```python
from build123d import *

# Parameters (mm, degrees)
BOSS_EXTRUDE1_DEPTH = 3
SKETCH3_W           = 4.2
SKETCH3_H           = 3.2
SKETCH3_W_2         = 3.2
SKETCH3_H_2         = 8.2
SKETCH3_W_3         = 8.2
CUT_EXTRUDE1_DEPTH  = 4


with BuildPart() as part:
    # Sketch1 → Boss-Extrude1 (new body)
    with BuildSketch(Plane.XY):
        Polygon((0, 52.125), (80, 52.125), (80, 3.175), (64, 3.175), (64, 15.625), (16, 15.625), (16, 3.175), (0, 3.175), align=None)
    extrude(amount=-BOSS_EXTRUDE1_DEPTH)

    # Sketch3 → Cut-Extrude1 (cut, through all)
    with BuildSketch(Plane.XY):
        with Locations((2, 50.625)):
            Rectangle(SKETCH3_W, SKETCH3_H)
        with Locations((1.5, 20.925)):
            Rectangle(SKETCH3_W_2, SKETCH3_H_2)
        with Locations((24, 17.125)):
            Rectangle(SKETCH3_W_3, SKETCH3_H)
        with Locations((40, 17.125)):
            Rectangle(SKETCH3_W_3, SKETCH3_H)
        with Locations((1.5, 36.925)):
            Rectangle(SKETCH3_W_2, SKETCH3_H_2)
        with Locations((40, 50.625)):
            Rectangle(SKETCH3_W_3, SKETCH3_H)
        with Locations((40, 42.425)):
            Rectangle(SKETCH3_W_3, SKETCH3_H)
        with Locations((24, 42.425)):
            Rectangle(SKETCH3_W_3, SKETCH3_H)
        with Locations((24, 50.625)):
            Rectangle(SKETCH3_W_3, SKETCH3_H)
        with Locations((56, 42.425)):
            Rectangle(SKETCH3_W_3, SKETCH3_H)
        with Locations((56, 17.125)):
            Rectangle(SKETCH3_W_3, SKETCH3_H)
        with Locations((78.5, 36.925)):
            Rectangle(SKETCH3_W_2, SKETCH3_H_2)
        with Locations((78, 50.625)):
            Rectangle(SKETCH3_W, SKETCH3_H)
        with Locations((78.5, 20.925)):
            Rectangle(SKETCH3_W_2, SKETCH3_H_2)
        with Locations((56, 50.625)):
            Rectangle(SKETCH3_W_3, SKETCH3_H)
        Polygon((76.9, 9.025), (76.9, 6.275), (67.9, 6.275), (67.9, 3.075), (80.1, 3.075), (80.1, 9.025), align=None)
        Polygon((3.1, 6.275), (3.1, 9.025), (-0.1, 9.025), (-0.1, 3.075), (12.1, 3.075), (12.1, 6.275), align=None)
    extrude(amount=-CUT_EXTRUDE1_DEPTH, mode=Mode.SUBTRACT)


solid = part.part
```
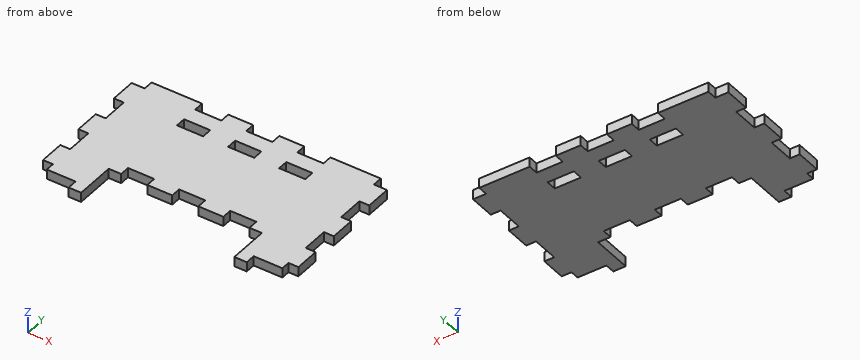
Read the model definition and answer for the solid it produces. Units are mm, in the model's axes. Give positions to 0.01 mm unless a question says otherwise; leave off trailing zeros. Order: outer loops, then holes, each group sorted by start corner. A loop starts at its lowest first (then second) coordinate and runs counter-clockwise, first axis right, second up. Notation, with made-up numbers: (45.5, 7) -> (52.5, 7) arc R25 cw to (52.5, 44) -> close; hole circle Ø7 at (-37.5, -17.75). An arc over 180 degrees is marked (long way). One line per item, written item: value. Start each with the question number.
(1) The part is cut by section D-D (z = -0.95). State how many separate pieces and enclosed holes the cut face has, and give its area (3 significant figures).
(2) Flat-ended cylindrical pins translate along their axes: P1, Ø0.9, axis at x = 2, z = -1, coming from the -Y side (3 decimals); P2, Ø1.5, axis at x = 24, z = -1, coming from the +Y side (3 decimals); P3, Ø0.9, axis at x = 8, z = -1.5, coming from the -Y side (3 decimals). Find the tip coordinate at first contact, or state that the pin passes through.
(3) The part is cut by section C-C (y = 10.5). Determine the outline of the cut face in (x, z).
(4) The part is cut by section A-A (y = 43). Determine the outline of the cut face in (x, z).
(5) Straight lines are drawn through the part: L1, parallel to Y at x = 43, z = -0.7 (3 decimals); L2, parallel to X at y = 42.5, z = -0.65; L3, parallel to Y at x = 35.5, z = -2.1 (3 decimals). For each, find the intervals that lie inside material, in ascending order.
(6) The part is cut by section B-B (x = 57). Determine the outline of the cut face in (y, z) (3 decimals).
Taken from the geometry:
1. separate pieces: 1
1. enclosed holes: 3
1. area: 2,870 mm^2
2. P1: y = 9.025
2. P2: y = 49.025
2. P3: y = 6.275
3. outline: (0, -3) -> (16, -3) -> (16, 0) -> (0, 0) -> close; (64, -3) -> (80, -3) -> (80, 0) -> (64, 0) -> close
4. outline: (0, -3) -> (19.9, -3) -> (19.9, 0) -> (0, 0) -> close; (28.1, -3) -> (35.9, -3) -> (35.9, 0) -> (28.1, 0) -> close; (44.1, -3) -> (51.9, -3) -> (51.9, 0) -> (44.1, 0) -> close; (60.1, -3) -> (80, -3) -> (80, 0) -> (60.1, 0) -> close
5. L1: 18.725 to 40.825, 44.025 to 49.025
5. L2: 0 to 19.9, 28.1 to 35.9, 44.1 to 51.9, 60.1 to 80
5. L3: 15.625 to 52.125
6. outline: (18.725, -3) -> (40.825, -3) -> (40.825, 0) -> (18.725, 0) -> close; (44.025, -3) -> (49.025, -3) -> (49.025, 0) -> (44.025, 0) -> close
